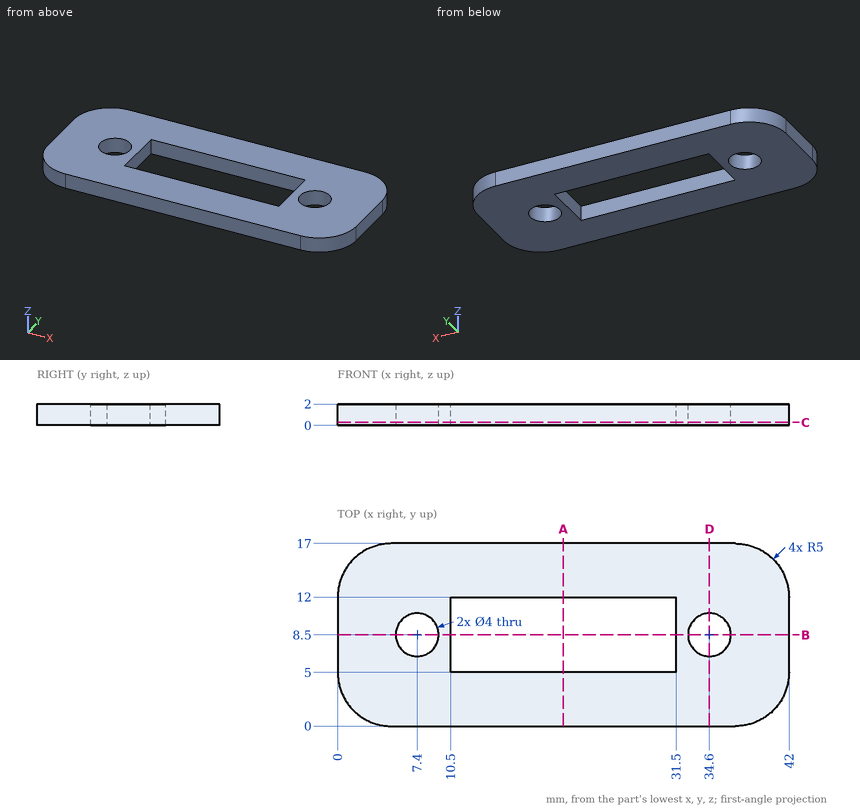
Geometry: see drawing. Coordinates: mm, zero at the bounding-box minimum. Round coordinates to 2 decimals unless told otherwise and drop trailing zeros. Loops run counter-clockwise (first coordinate to the right, second up) from the corner with the lowest first, then second, coordinate; pieces in that order, holes last. Notation, with made-up numbers: M 54,85.25 L 92,85.25 A12 cw 92,107.25 Z; hole C 40,66 d8. An arc over 180 degrees is marked long. Use a Markdown table: item, result. Add a question column.
1. Cut plane D-D, the plane x = 34.6. Output: boundary loops of the cut face in (y, z).
2. Ray query, line 1 along Y through (x, z) = (21, 1.75); line 2 along Y through (x, z) = (34.6, 1.55); line 3 along X through (y, z) = (7.5, 0.7). Return the intervals inside material, ascending. Write a range as [from, to].
3. Cut plane B-B, the plane y = 8.5. Output: boundary loops of the cut face in (x, z), and give its area (3 significant figures).
4. Cut plane A-A, the plane x = 21. Output: boundary loops of the cut face in (y, z).
5. Cut plane C-C, the plane z = 0.3. Output: boundary loops of the cut face in (x, y).
Solution:
| question | item | result |
|---|---|---|
| 1 | outline | M 0,0 L 6.5,0 L 6.5,2 L 0,2 Z; M 10.5,0 L 17,0 L 17,2 L 10.5,2 Z |
| 2 | line 1 | y = [0, 5], [12, 17] |
| 2 | line 2 | y = [0, 6.5], [10.5, 17] |
| 2 | line 3 | x = [0, 5.67], [9.13, 10.5], [31.5, 32.87], [36.33, 42] |
| 3 | outline | M 0,0 L 5.4,0 L 5.4,2 L 0,2 Z; M 9.4,0 L 10.5,0 L 10.5,2 L 9.4,2 Z; M 31.5,0 L 32.6,0 L 32.6,2 L 31.5,2 Z; M 36.6,0 L 42,0 L 42,2 L 36.6,2 Z |
| 3 | area | 26.0 mm2 |
| 4 | outline | M 0,0 L 5,0 L 5,2 L 0,2 Z; M 12,0 L 17,0 L 17,2 L 12,2 Z |
| 5 | outline | M 0,5 A5 ccw 5,0 L 37,0 A5 ccw 42,5 L 42,12 A5 ccw 37,17 L 5,17 A5 ccw 0,12 Z; hole C 7.4,8.5 d4; hole M 10.5,5 L 31.5,5 L 31.5,12 L 10.5,12 Z; hole C 34.6,8.5 d4 |
